Read the model definition and answer for the solid it produces. Units are mm, in the model's axes. Face numbers are marked on the shaded views. Give positions to 0.01 mm unless a question says otherwise; leave off trailing zeros. Order: outer loops, then holes, each group sorted by start corner. A loop starts at its lowest first (then second) coordinate and runs counter-clockwise, first axis right, second up. Notation, with made-up numbers: (80.5, 12.25) - (116.5, 12.25) arc R24 ccw to (116.5, 37.25) - close; hole circle Ø8 at (56.25, -16). An arc over 180 degrees is marked (long way). Use a Markdown table: item, result. Add a question column.
1. A cutting plane is placed at B-B on z = -22.5. Determine the outline of the cut face in (x, y), and give its area (3 significant figures).
2. A cutting plane is placed at A-A on x = -16.25. Determine the outline of the cut face in (y, z).
3. Consider L1, parallel to Y at x = -28, z = -16. Determine where the line is inside the solid, lowest interval first.
4. Flat-ended cylindrical pins translate along their axes: P1, Ø0.5, axis at x = -24.5, y = -5.5, coming from the +Z side; P2, Ø5, axis at x = -25, z = -4.5, coming from the -Y side. Find the tip coordinate at first contact, or state that the pin passes through.
5. For a pull along X with two mould halves and no side action, classify the marked faces 1 and 2 as released by +X, released by -X, zero draft, split by the parting line, or undercut.
6. A cutting plane is placed at C-C on x = -26.5. Determine the outline of the cut face in (y, z), and give its area (3 significant figures).
7. A cutting plane is placed at D-D on x = -12.5. Determine the outline of the cut face in (y, z), and give its area (3 significant figures).
```python
from build123d import *

# Parameters (mm, degrees)
F0_W     = 28.651202
F0_H     = 54.254404
F1_DEPTH = 4.572
F2_R     = 1.777274
F2_W     = 18.440403
F2_H     = 14.630441
F3_DEPTH = 1.016


with BuildPart() as f1:
    # F0 (on Front) → F1 (new body)
    with BuildSketch(Plane.XZ):
        with Locations((-20.421601, -6.5532)):
            Rectangle(F0_W, F0_H)
    extrude(amount=F1_DEPTH)

    # F2 (on face) → F3 (join)
    with BuildSketch(Plane.XZ.offset(4.572)):
        with Locations((-11.2776, -4.7244)):
            Circle(F2_R)
        with Locations((-23.0886, 8.68678)):
            Rectangle(F2_W, F2_H)
        Polygon((-29.184598, 8.68678), (-29.184598, 13.146272), (-23.0886, 13.146272), (-16.992602, 13.146272), (-16.992602, 8.68678), (-16.992602, 4.227289), (-23.0886, 4.227289), (-29.184598, 4.227289), align=None, mode=Mode.SUBTRACT)
    extrude(amount=F3_DEPTH)


solid = f1.part
```
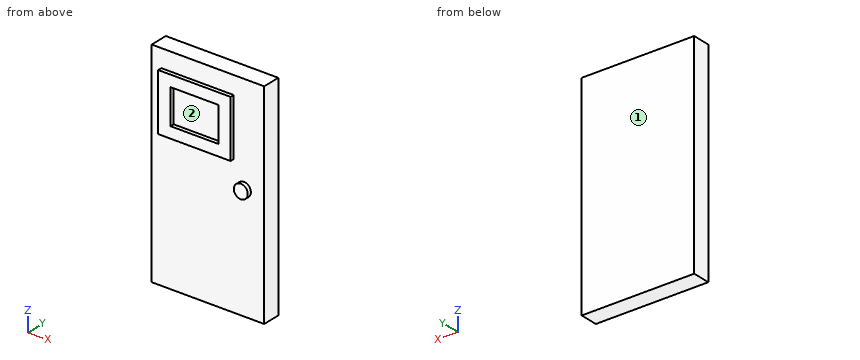
Output values:
| question | item | result |
|---|---|---|
| 1 | outline | (-34.75, -4.57) - (-6.1, -4.57) - (-6.1, 0) - (-34.75, 0) - close |
| 1 | area | 131 mm² |
| 2 | outline | (-5.59, 1.37) - (-4.57, 1.37) - (-4.57, -33.68) - (0, -33.68) - (0, 20.57) - (-4.57, 20.57) - (-4.57, 16) - (-5.59, 16) - close |
| 3 | L1 | -4.57 to 0 |
| 4 | P1 | z = 16 |
| 4 | P2 | y = -4.57 |
| 5 | face 1 | zero draft |
| 5 | face 2 | undercut |
| 6 | outline | (-5.59, 1.37) - (-4.57, 1.37) - (-4.57, -33.68) - (0, -33.68) - (0, 20.57) - (-4.57, 20.57) - (-4.57, 16) - (-5.59, 16) - (-5.59, 13.15) - (-4.57, 13.15) - (-4.57, 4.23) - (-5.59, 4.23) - close |
| 6 | area | 254 mm² |
| 7 | outline | (-5.59, -6.01) - (-4.57, -6.01) - (-4.57, -33.68) - (0, -33.68) - (0, 20.57) - (-4.57, 20.57) - (-4.57, -3.43) - (-5.59, -3.43) - close |
| 7 | area | 251 mm² |
